Could you check a few things on this model? Use its own coordinates, in mm. Coordinates: 2 decimals unless noted, no trailing zeros. Loops run counter-clockwise (first coordinate to the right, second up) from the corner with the lowest first, then second, coordinate; pieces in that order, holes last. Notation, with made-up numbers: M 45.5,7 L 103.5,7 A28 ccw 103.5,28 Z; hole C 70.25,18 d7. An arc over 180 degrees is marked long. Return JSON: item names as keys, results as strings. Group by question number.
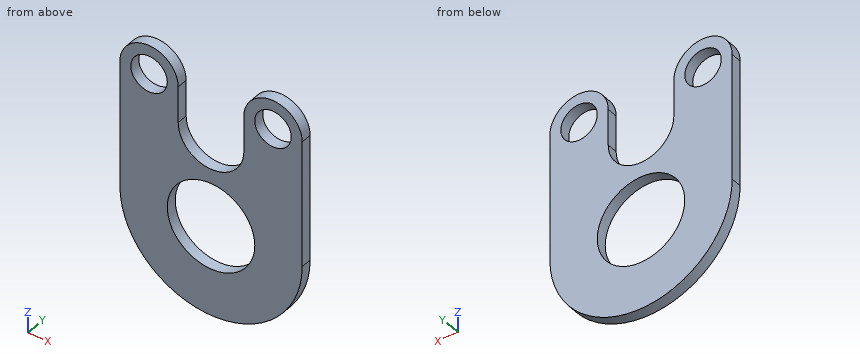
from build123d import *

# Parameters (mm, degrees)
SKETCH1_R           = 12
SKETCH1_R_2         = 5
BOSS_EXTRUDE2_DEPTH = 1.5


with BuildPart() as part:
    # Sketch1 → Boss-Extrude2 (new body, symmetric)
    with BuildSketch(Plane(origin=(0, 0, 0), x_dir=(1, 0, 0), z_dir=(0, 1, 0))):
        with BuildLine():
            Line((-25, 0), (-25, -35))
            ThreePointArc((-25, -35), (-17, -43), (-9, -35))
            Line((-9, -35), (-9, -25))
            ThreePointArc((-9, -25), (0, -16), (9, -25))
            Line((9, -25), (9, -35))
            ThreePointArc((9, -35), (17, -43), (25, -35))
            Line((25, -35), (25, 0))
            ThreePointArc((25, 0), (0, 25), (-25, 0))
        make_face()
        Circle(SKETCH1_R, mode=Mode.SUBTRACT)
        with Locations((17, -35)):
            Circle(SKETCH1_R_2, mode=Mode.SUBTRACT)
        with Locations((-17, -35)):
            Circle(SKETCH1_R_2, mode=Mode.SUBTRACT)
    extrude(amount=BOSS_EXTRUDE2_DEPTH, both=True)


solid = part.part
(1) If I drill on L1, parallel to X at y = 0.65, z = 35; L2, parallel to X at y = 1.2, z = 32; L3, parallel to X at y = 0.15, z = 0, over which ranges is the centre line in solid material (lowest first)? Write a range as [from, to].
(2) Imagine slicing it at C-C, the plane x = 17. Write out the boundary of the cut face in (y, z), then the cut area to 3 significant figures.
(3) Imagine slicing it at B-B, the plane z = 26. Write out the boundary of the cut face in (x, y), then the cut area to 3 significant figures.
(4) Imagine slicing it at A-A, the plane y = -0.2. Write out the boundary of the cut face in (x, z).
(5) Will these pins go through, and if not, where does the flat tip stop? P1, Ø9, axis at x = -17, z = 35, coming from the +Y side; P2, Ø1, axis at y = 1, z = -5, coming from the +X side.
Checks:
{
 "1": {"L1": "[-25, -22], [-12, -9], [9, 12], [22, 25]", "L2": "[-25, -21], [-13, -9], [9, 13], [21, 25]", "L3": "[-25, -12], [12, 25]"},
 "2": {"outline": "M -1.5,-18.33 L 1.5,-18.33 L 1.5,30 L -1.5,30 Z; M -1.5,40 L 1.5,40 L 1.5,43 L -1.5,43 Z", "area": "154 mm²"},
 "3": {"outline": "M -25,-1.5 L -9,-1.5 L -9,1.5 L -25,1.5 Z; M 9,-1.5 L 25,-1.5 L 25,1.5 L 9,1.5 Z", "area": "96.0 mm²"},
 "4": {"outline": "M -25,0 A25 ccw 25,0 L 25,35 A8 ccw 9,35 L 9,25 A9 cw -9,25 L -9,35 A8 ccw -25,35 Z; hole C -17,35 d10; hole C 0,0 d24; hole C 17,35 d10"},
 "5": {"P1": "through", "P2": "x = 24.59"}
}
